Build history of the part. All positions in model axes, mm. A direction names the side the tool comes from. Round coordinates to 2 decimals unless told otherwise and drop trailing zeros. Write each loop counter-clockwise with the first axis right and the second up, starting at its lowest first coordinate (ties: lowest second). Pieces come first, ordered by that corner, then holes. Notation, with made-up numbers: M 21.25,37.5 L 33.25,37.5 A23 ccw 33.25,63.5 Z; hole C -39.5,-8 d2. An arc over 180 degrees is marked long. Write item = value, one per line.
from build123d import *

# Parameters (mm, degrees)
SKETCH_1_R      = 4
SKETCH_1_R_2    = 2.5
EXTRUDE_1_DEPTH = 5


with BuildPart() as part:
    # 草图1 → 凸台-拉伸1 (new body)
    with BuildSketch(Plane(origin=(0, 0, 0), x_dir=(0, 0, -1), z_dir=(1, 0, 0))):
        Polygon((-62.127361451, 56.787762609), (-75.627361451, 56.787762609), (-75.627361451, 53.787762609), (-74.377361451, 53.787762609), (-74.377361451, 50.787762609), (-75.627361451, 50.787762609), (-75.627361451, 48.787762609), (-78.627361451, 48.787762609), (-78.627361451, 50.787762609), (-79.877361451, 50.787762609), (-79.877361451, 53.787762609), (-78.627361451, 53.787762609), (-78.627361451, 56.787762609), (-92.127361451, 56.787762609), (-92.127361451, 46.787762609), (-87.127361451, 46.787762609), (-87.127361451, 26.787762609), (-92.127361451, 26.787762609), (-92.127361451, 11.787762609), (-87.127361451, 11.787762609), (-87.127361451, -8.212237391), (-92.127361451, -8.212237391), (-92.127361451, -18.212237391), (-62.127361451, -18.212237391), (-62.127361451, -23.212237391), (-22.127361451, -23.212237391), (-22.127361451, -18.212237391), (12.872638549, -18.212237391), (12.872638549, -8.212237391), (7.872638549, -8.212237391), (7.872638549, 11.787762609), (12.872638549, 11.787762609), (12.872638549, 26.787762609), (7.872638549, 26.787762609), (7.872638549, 46.787762609), (12.872638549, 46.787762609), (12.872638549, 56.787762609), (-3.127361451, 56.787762609), (-3.127361451, 53.787762609), (-1.877361451, 53.787762609), (-1.877361451, 50.787762609), (-3.127361451, 50.787762609), (-3.127361451, 48.787762609), (-6.127361451, 48.787762609), (-6.127361451, 50.787762609), (-7.377361451, 50.787762609), (-7.377361451, 53.787762609), (-6.127361451, 53.787762609), (-6.127361451, 56.787762609), (-22.127361451, 56.787762609), (-22.127361451, 61.787762609), (-62.127361451, 61.787762609), align=None)
        with Locations((-39.627361451, 19.287762609)):
            Circle(SKETCH_1_R, mode=Mode.SUBTRACT)
        with Locations((-39.627361451, 37.787762609)):
            Circle(SKETCH_1_R_2, mode=Mode.SUBTRACT)
        with Locations((-39.627361451, 0.787762609)):
            Circle(SKETCH_1_R_2, mode=Mode.SUBTRACT)
        with Locations((-26.627361451, 49.287762609)):
            Circle(SKETCH_1_R, mode=Mode.SUBTRACT)
        with Locations((-26.627361451, -10.712237391)):
            Circle(SKETCH_1_R, mode=Mode.SUBTRACT)
    extrude(amount=EXTRUDE_1_DEPTH)


solid = part.part
1. Band-saw the part on C-C (z = 81.5). List the corners of the cut face in (x, y), plus the area to 3 significant figures.
Responses:
outline = M 0,-18.21 L 5,-18.21 L 5,56.79 L 0,56.79 Z
area = 375 mm²
2. Mould opens along Y. For faces 4 (the face through (2, 61.788, 42)), 5 (the face through (2, 52, -12.873)), 6 (the face through (2, 37, -7.873)) say: pulls with the +Y half, pulls with the -Y half, needs draft (parallel to the pull), parting line crosses it, or undercut.
Responses:
face_4 = pulls with the +Y half
face_5 = needs draft
face_6 = undercut
3. Band-saw the part on B-B (x = 2.1). Count the separate pieces of the cut face and the enclosed holes in it, plus the area to 3 significant figures.
Responses:
separate_pieces = 1
enclosed_holes = 5
area = 7,620 mm²
4. Tool access for faces 1 (the face through (2, 52, 79.877)), 2 (the face through (2, 59, 62.127)), 3 (the face through (2, 48.788, 5)): list every direction of +Z, -Z, +X, -X, +Y, -Y with a clear straight run to the whole face (end or side of a thin tool).
Responses:
face_1 = +X, -X
face_2 = +Z, +X, -X, +Y
face_3 = +X, -X, +Y
5. Band-saw the part on D-D (y = 2). List the corners of the cut face in (x, z).
Responses:
outline = M 0,-7.87 L 5,-7.87 L 5,37.44 L 0,37.44 Z; M 0,41.81 L 5,41.81 L 5,87.13 L 0,87.13 Z
6. Band-saw the part on A-A (y = -13). List the corners of the cut face in (x, z), plus the area to 3 significant figures.
Responses:
outline = M 0,-12.87 L 5,-12.87 L 5,23.35 L 0,23.35 Z; M 0,29.91 L 5,29.91 L 5,92.13 L 0,92.13 Z
area = 492 mm²
7. Probe probe 1 along Z at (x, y) = (2.85, 52); probe 2 along Y at (x, z) = (0.8, 2.5); probe 3 along Y at (x, z) = (2.35, 41). List the from-to ranges inside material, lowest first.
Responses:
probe_1 = -12.87 to 1.88, 7.38 to 23.69, 29.57 to 74.38, 79.88 to 92.13
probe_2 = -18.21 to 50.79, 53.79 to 56.79
probe_3 = -23.21 to -1.3, 2.88 to 15.53, 23.04 to 35.7, 39.88 to 61.79
8. Flat gauge pins, fed straight in: pin 1 (2.5 mm diameter, centred on x = 3, z = 17, fed in from +Y); pin 2 (2.5 mm diameter, centred on x = 2.5, z = 77, fed in from +Y); pin 3 (1.5 mm diameter, centred on x = 2, y = 32.5, fed in from +Z). Where does each tip first touch, or does it go through?
Responses:
pin_1 = 56.79
pin_2 = 48.79
pin_3 = 87.13
